```python
from build123d import *

# Parameters (mm, degrees)
F1_DEPTH  = 76.2
F2_W      = 45.2374
F2_H      = 57.912
F3_DEPTH  = 38.1
F4_W      = 0.9906
F4_H      = 1.6002
F5_DEPTH  = 25.4
F6_W      = 0.7274897046
F6_H      = 0.9906
F7_DEPTH  = 2.54
F8_W      = 1.1825356632
F8_H      = 1.4120219275
F9_DEPTH  = 25.4
F10_W     = 0.5234003049
F10_H     = 1.1825356632
F11_DEPTH = 2.54
F13_DEPTH = 12.7
F14_W     = 17.834963277
F14_H     = 73.4775259625
F15_DEPTH = 12.7
F16_W     = 18.2606615126
F16_H     = 72.5786741823
F17_DEPTH = 10.16


with BuildPart() as f1:
    # F0 (on Front) → F1 (new body)
    with BuildSketch(Plane.XZ):
        Polygon((8.871205765, 56.1352521181), (-41.928794235, 56.1352521181), (-53.7675097585, 44.2965365946), (-74.4852647185, 44.2965365946), (-80.3059687692, 47.2815136811), (-81.8367265829, 44.2965365946), (-74.4852647185, 34.8938606037), (-53.7675097585, 27.7223307639), (-53.7675097585, 7.7938223258), (-43.7045991421, 2.6637113187), (-36.7986820638, 13.1148345131), (2.4190642002, 13.1148345131), (6.4126392826, 3.4529594705), (21.2110355496, 9.5696300268), (21.2110355496, 24.1707172245), (40.7449230552, 29.4981393963), (51.1220302522, 38.4206696416), (49.2293350399, 43.5072891414), (40.7449230552, 40.3502993286), (21.2110355496, 44.2965365946), align=None)
    extrude(amount=F1_DEPTH)

    # F2 (on face) → F3 (cut)
    with BuildSketch(Plane.XY.offset(56.1352521181)):
        with Locations((-16.5863556839, -31.4929929974)):
            Rectangle(F2_W, F2_H)
    extrude(amount=-F3_DEPTH, mode=Mode.SUBTRACT)

    # F4 (on face) → F5 (join)
    with BuildSketch(Plane(origin=(57.4622590525, 0, 21.381301), x_dir=(0, 1, 0), z_dir=(0.9372218761, 0, 0.3487336448))):
        with Locations((-51.2663501552, 20.6706811054)):
            Rectangle(F4_W, F4_H)
    extrude(amount=F5_DEPTH)

    # F6 (on face) → F7 (join)
    with BuildSketch(Plane(origin=(-7.487583751, 0, 20.1228857485), x_dir=(0.9372218761, 0, 0.3487336448), z_dir=(-0.3487336448, 0, 0.9372218761))):
        with Locations((86.3475204084, -51.2663501552)):
            Rectangle(F6_W, F6_H)
    extrude(amount=F7_DEPTH)

    # F8 (on face) → F9 (join)
    with BuildSketch(Plane(origin=(-82.7823804145, 0, 42.4525120249), x_dir=(0, -1, 0), z_dir=(-0.8898174224, 0, 0.4563167263))):
        with Locations((28.4478189424, 4.0023266338)):
            Rectangle(F8_W, F8_H)
    extrude(amount=F9_DEPTH)

    # F10 (on face) → F11 (join)
    with BuildSketch(Plane(origin=(2.1484931989, 0, 4.1895608251), x_dir=(0.8898174224, 0, -0.4563167263), z_dir=(0.4563167263, 0, 0.8898174224))):
        with Locations((-118.1712955227, -28.4478189424)):
            Rectangle(F10_W, F10_H)
    extrude(amount=F11_DEPTH)

    # F12 (on face) → F13 (cut)
    with BuildSketch(Plane.XZ.offset(76.2)):
        Polygon((-35.403739661, 34.8885591957), (-37.6328639686, 38.2322445512), (-40.683247149, 32.4834473431), (-25.0793676823, 25.9133949876), (-9.9447797984, 30.0196781754), (-9.9447797984, 38.3495688438), (-12.0826530857, 34.8885591957), (-13.6990956962, 37.3132223095), (-17.336089164, 34.8885591957), (-18.2746686041, 38.3495688438), (-21.5596966445, 34.8885591957), (-26.9956346343, 34.8885591957), (-29.3029751629, 38.3495688438), (-30.6326299647, 34.8885591957), (-32.9399704933, 38.3495688438), align=None)
        Polygon((-30.241554603, 49.1432286799), (-32.9399704933, 52.5455772877), (-35.403739661, 51.0203875601), (-33.6285175147, 48.1527196821), align=None)
        Polygon((-8.1849442795, 51.0203875601), (-10.8833583072, 51.0203875601), (-13.6990956962, 49.1432286799), (-6.9335046121, 49.1432286799), align=None)
    extrude(amount=-F13_DEPTH, mode=Mode.SUBTRACT)

    # F14 (on face) → F15 (cut)
    with BuildSketch(Plane(origin=(9.429613944, 0, 46.6766201788), x_dir=(0.9801980455, 0, -0.198019675), z_dir=(0.198019675, 0, 0.9801980455))):
        with Locations((21.7831684276, -37.9125081236)):
            Rectangle(F14_W, F14_H)
    extrude(amount=-F15_DEPTH, mode=Mode.SUBTRACT)

    # F16 (on face) → F17 (cut)
    with BuildSketch(Plane.XY.offset(44.2965365946)):
        with Locations((-64.177474007, -38.1315993145)):
            Rectangle(F16_W, F16_H)
    extrude(amount=-F17_DEPTH, mode=Mode.SUBTRACT)


solid = f1.part
```
Source: CAD feature listing. Evaluate the final solid. Frame: model axes, mm. A direction names the side the tool comes from. Give positions to 0.01 mm unless a question says otherwise; leave off trailing zeros. Order: outer loops, then holes, each group sorted by start corner. A loop starts at its lowest first (then second) coordinate and runs counter-clockwise, first axis right, second up. Notation, with made-up numbers: (17.25, -6.5) -> (44.25, -6.5) arc R22 cw to (44.25, 15.5) -> close; hole circle Ø10 at (32.5, 63.5). An arc over 180 degrees is marked (long way). Use a Markdown table: item, result.
Q1. First-contact query: P1, Ø10, axis at x = 66.5, z = 43.5, coming from the +Y side; P2, Ø10, axis at x = -24, y = -8.5, coming from the -Z side; P3, Ø5.5, axis at x = -9, y = -70.5, coming from the +Z side. Flat tips, straight axial feed; report the tip coordinate or a pass-through.
A:
| item | result |
|---|---|
| P1 | y = -50.77 |
| P2 | z = 13.11 |
| P3 | z = 56.14 |
Q2. Section A-A (y = -57.5). State how many separate pieces and enclosed holes the cut face has, and give its area (3 significant figures).
A:
| item | result |
|---|---|
| separate pieces | 3 |
| enclosed holes | 0 |
| area | 1,880 mm^2 |
Q3. Access query for faces 1 (the face through (6.032, -32, 37)), 2 (the face through (45.861, -37.567, 33.897)), 3 (the face through (-54.87, -37.92, 44.297)), 4 (the face through (-24, -70, 34.889)). Directions: +Z, -Z, +X, -X, +Y, -Y. A direction counts if a zero-diameter tool reaches every point of the face in a straight line with its end or side. Return the directions, or none.
A:
| item | result |
|---|---|
| face 1 | +Z |
| face 2 | -Z, +X, +Y, -Y |
| face 3 | +Z, +Y, -Y |
| face 4 | -Y |
Q4. Section B-B (x = -70.5). Return the cut outline in (y, z), and give its area (3 significant figures).
A:
| item | result |
|---|---|
| outline | (-76.2, 33.51) -> (0, 33.51) -> (0, 44.3) -> (-1.84, 44.3) -> (-1.84, 34.14) -> (-74.42, 34.14) -> (-74.42, 44.3) -> (-76.2, 44.3) -> close |
| area | 84.2 mm^2 |
Q5. Material intervals for line 1 (Y direction, x = -32, z = 45); line 2 (Y direction, x = -66, z = 43); line 3 (X direction, y = -24.5, z = 44), sorted ascending. Write a range as [from, to].
A:
| item | result |
|---|---|
| line 1 | [-76.2, -60.45], [-2.54, 0] |
| line 2 | [-76.2, -74.42], [-1.84, 0] |
| line 3 | [-81.6, -73.31], [-55.05, -39.21], [6.03, 22.01] |
Q6. Pull-direction query (X, two-part tool) for faces 5 (the face through (45.047, -37.567, 41.951)), 6 (the face through (-48.806, -37.567, 5.265)), 7 (the face through (-73.308, -39, 39)), 8 (the face through (62, -50.771, 45)); classes: +X half, -X half, draft (parallel to the pull), parting line (faces both ways), or undercut.
A:
| item | result |
|---|---|
| face 5 | undercut |
| face 6 | -X half |
| face 7 | undercut |
| face 8 | draft |
Q7. Section C-C (z = 15). Return the cut outline in (x, y).
A:
| item | result |
|---|---|
| outline | (-53.77, -76.2) -> (21.21, -76.2) -> (21.21, 0) -> (-53.77, 0) -> close |
Q8. Section D-D (x = -91). Return the cut outline in (y, z).
A:
| item | result |
|---|---|
| outline | (-29.04, 50.37) -> (-27.86, 50.37) -> (-27.86, 51.96) -> (-29.04, 51.96) -> close |
